```python
from build123d import *

# Parameters (mm, degrees)
F0_R     = 2.25
F1_DEPTH = 1
F2_SIZE  = 7.5
F3_R     = 3.25
F4_DEPTH = 2


# Not quite as in the source:
# - a feature names something its author has since deleted; it is built from what else it names


with BuildPart() as f1:
    # F0 (on Front) → F1 (new body, symmetric)
    with BuildSketch(Plane.XZ):
        Polygon((226.3, 155), (226.3, 188), (-226.3, 188), (-226.3, 155), (-259.3, 155), (-259.3, -155), (-226.3, -155), (-226.3, -188), (226.3, -188), (226.3, -155), (259.3, -155), (259.3, 155), align=None)
        with BuildLine():
            ThreePointArc((129.1982753492, -109.35), (126.3, -121.35), (123.4017246508, -109.35))
            Line((123.4017246508, -109.35), (129.1982753492, -109.35))
        make_face(mode=Mode.SUBTRACT)
        with Locations((146.3, -115)):
            Circle(F0_R, mode=Mode.SUBTRACT)
        with BuildLine():
            Line((154.55, -104.5), (178.05, -104.5))
            ThreePointArc((178.05, -104.5), (179.817766953, -105.232233047), (180.55, -107))
            Line((180.55, -107), (180.55, -123))
            ThreePointArc((180.55, -123), (179.817766953, -124.767766953), (178.05, -125.5))
            Line((178.05, -125.5), (154.55, -125.5))
            ThreePointArc((154.55, -125.5), (152.782233047, -124.767766953), (152.05, -123))
            Line((152.05, -123), (152.05, -107))
            ThreePointArc((152.05, -107), (152.782233047, -105.232233047), (154.55, -104.5))
        make_face(mode=Mode.SUBTRACT)
        with Locations((186.3, -115)):
            Circle(F0_R, mode=Mode.SUBTRACT)
    extrude(amount=F1_DEPTH, both=True)

    # F2
    f2_edges = [f1.edges().sort_by_distance(p)[0] for p in [
        (226.3, 0, 188),
        (259.3, 0, 155),
        (259.3, 0, -155),
        (226.3, 0, -188),
        (-226.3, 0, 188),
        (-259.3, 0, 155),
        (-259.3, 0, -155),
        (-226.3, 0, -188),
    ]]
    chamfer(f2_edges, length=F2_SIZE)

    # F3 (on face) → F4 (cut, through all)
    with BuildSketch(Plane.XZ.offset(1)):
        Polygon((-228.55, -152.75), (-228.55, -155), (-226.3, -155), (-226.3, -157.25), (-224.05, -157.25), (-224.05, -152.75), align=None)
        Polygon((226.3, -155), (228.55, -155), (228.55, -152.75), (224.05, -152.75), (224.05, -157.25), (226.3, -157.25), align=None)
        with Locations((-236.6, 149.1)):
            Circle(F3_R)
        with Locations((-236.6, 72.9)):
            Circle(F3_R)
        with Locations((-236.6, 34.3)):
            Circle(F3_R)
        with Locations((-236.6, -112.4)):
            Circle(F3_R)
        with Locations((236.6, -112.4)):
            Circle(F3_R)
        with Locations((236.6, 34.3)):
            Circle(F3_R)
        with Locations((236.6, 72.9)):
            Circle(F3_R)
        with Locations((236.6, 149.1)):
            Circle(F3_R)
        Polygon((226.3, 155), (226.3, 157.25), (224.05, 157.25), (224.05, 152.75), (228.55, 152.75), (228.55, 155), align=None)
        Polygon((-224.05, 152.75), (-224.05, 157.25), (-226.3, 157.25), (-226.3, 155), (-228.55, 155), (-228.55, 152.75), align=None)
    extrude(amount=-F4_DEPTH, mode=Mode.SUBTRACT)


solid = f1.part
```
Source: CAD feature listing. Evaluate the final solid. Frame: model axes, mm. Round coordinates to 2 decimals unless told otherwise and drop trailing zeros. Loops run counter-clockwise (first coordinate to the right, second up) from the corner with the lowest first, then second, coordinate; pieces in that order, holes last. Notation, with made-up numbers: M 40.5,-40 L 85.5,-40 A20 cw 85.5,-19 Z; hole C 38,8 d5. An arc over 180 degrees is marked long. Use a Markdown table: item, result. Add a question column.
1. Section query B-B on z = 164.5. Return the cut outline in (x, y), then the cut area to 3 significant figures.
2. Mould query, pull axis Z, two halves, no side actions, for faces 1 (the flat face through (-4, 1, 3)), 2 (the cylindrical face through (126.537, -0.014, -121.346)). Classes: pulls with the +Z half, pulls with the -Z half, needs draft (parallel to the pull), parting line crosses it, or undercut.
3. Contact query for flat-ended pins moving along their axis: P1, Ø1, axis at x = 225.5, y = 0, coming from the -Z side; P2, Ø7.5, axis at x = 126.3, z = -115, coming from the +Y side; P3, Ø0.6, axis at y = 0, z = -154.5, coming from the -X side; P4, Ø0.6, axis at x = 244, y = 0, coming from the -Z side. Output: stop coordinate, or through.
4. Line query: line 1 (Z direction, x = -236.6, y = -0.3); line 2 (X direction, y = 0.8, z = 33.5); line 3 (X direction, y = -0.1, z = 149.1). Output: solid intervals per line, ascending.
5. Section query A-A on y = -0.55. Give the number of separate pieces and of enclosed holes in the cut face, then the cut area to 3 significant figures.
Reported:
| question | item | result |
|---|---|---|
| 1 | outline | M -226.3,-1 L 226.3,-1 L 226.3,1 L -226.3,1 Z |
| 1 | area | 905 mm² |
| 2 | face 1 | needs draft |
| 2 | face 2 | undercut |
| 3 | P1 | stops at z = -181.8 |
| 3 | P2 | passes through |
| 3 | P3 | stops at x = -252.6 |
| 3 | P4 | stops at z = -155 |
| 4 | line 1 | z = -155 to -115.65, -109.15 to 31.05, 37.55 to 69.65, 76.15 to 145.85, 152.35 to 155 |
| 4 | line 2 | x = -259.3 to -239.75, -233.45 to 233.45, 239.75 to 259.3 |
| 4 | line 3 | x = -257.7 to -239.85, -233.35 to 233.35, 239.85 to 257.7 |
| 5 | separate pieces | 1 |
| 5 | enclosed holes | 12 |
| 5 | area | 189,000 mm² |
